```python
from build123d import *

# Parameters (mm, degrees)
SKETCH_R        = 6.2
SKETCH_R_2      = 4
PAD_DEPTH       = 8
PAD001_DEPTH    = 3
FILLET_R        = 1.5
FILLET001_R     = 1
SKETCH002_W     = 2
SKETCH002_H     = 10
SKETCH002_W_2   = 10
SKETCH002_H_2   = 2
PAD002_DEPTH    = 2
CHAMFER_SIZE    = 1.99
SKETCH003_R     = 6.2
SKETCH003_R_2   = 5.59
POCKET_DEPTH    = 3
SKETCH004_W     = 1
SKETCH004_H     = 14
POCKET001_DEPTH = 6
CHAMFER001_SIZE = 0.59
CHAMFER004_SIZE = 1


with BuildPart() as part:
    # Sketch → Pad (new body)
    with BuildSketch(Plane.XY):
        with Locations((15, 15)):
            Circle(SKETCH_R)
        with Locations((15, 15)):
            Circle(SKETCH_R_2, mode=Mode.SUBTRACT)
    extrude(amount=PAD_DEPTH)

    # Sketch001 (on Face3 of Pad) → Pad001 (join)
    with BuildSketch(Plane(origin=(0, 0, 0), x_dir=(1, 0, 0), z_dir=(0, 0, -1))):
        with BuildLine():
            Line((0, -28.504743), (0, 0))
            Line((0, 0), (28.504743, 0))
            ThreePointArc((30.002374, -1.584264), (29.594788, -0.469562), (28.504743, 0))
            ThreePointArc((1.584264, -30.002374), (21.216341, -21.216341), (30.002374, -1.584264))
            ThreePointArc((0, -28.504743), (0.469562, -29.594788), (1.584264, -30.002374))
        make_face()
    extrude(amount=PAD001_DEPTH)

    # Fillet
    fillet_edges = [part.edges().sort_by_distance(p)[0] for p in [
        (0, 0, -1.5),
    ]]
    fillet(fillet_edges, radius=FILLET_R)

    # Fillet001
    fillet001_edges = [part.edges().sort_by_distance(p)[0] for p in [
        (0, 15.002371, -3),
        (0.43934, 0.43934, -3),
        (0.469562, 29.594788, -3),
        (15.002371, 0, -3),
        (21.216341, 21.216341, -3),
        (29.594788, 0.469562, -3),
    ]]
    fillet(fillet001_edges, radius=FILLET001_R)

    # Sketch002 (on Face4 of Fillet001) → Pad002 (join)
    with BuildSketch(Plane.XY):
        with Locations((6, 15)):
            Rectangle(SKETCH002_W, SKETCH002_H)
        with Locations((15, 6)):
            Rectangle(SKETCH002_W_2, SKETCH002_H_2)
    extrude(amount=PAD002_DEPTH)

    # Chamfer
    chamfer_edges = [part.edges().sort_by_distance(p)[0] for p in [
        (15, 5, 0),
        (5, 15, 0),
    ]]
    chamfer(chamfer_edges, length=CHAMFER_SIZE)

    # Sketch003 → Pocket (cut)
    with BuildSketch(Plane.XY):
        with Locations((15, 15)):
            Circle(SKETCH003_R)
        with Locations((15, 15)):
            Circle(SKETCH003_R_2, mode=Mode.SUBTRACT)
    extrude(amount=POCKET_DEPTH, mode=Mode.SUBTRACT)

    # Sketch004 (on Face32 of Pocket) → Pocket001 (cut)
    with BuildSketch(Plane.XY.offset(8)):
        with Locations((15, 15)):
            Rectangle(SKETCH004_W, SKETCH004_H)
    extrude(amount=-POCKET001_DEPTH, mode=Mode.SUBTRACT)

    # Chamfer001
    chamfer001_edges = [part.edges().sort_by_distance(p)[0] for p in [
        (19.557412, 19.20357, 8),
        (19.125718, 18.77181, 3),
        (9.41, 15, 3),
        (9.41, 15, 0),
        (8.8, 15, 8),
    ]]
    chamfer(chamfer001_edges, length=CHAMFER001_SIZE)

    # Chamfer004
    chamfer004_edges = [part.edges().sort_by_distance(p)[0] for p in [
        (11, 15, 0),
    ]]
    chamfer(chamfer004_edges, length=CHAMFER004_SIZE)


solid = part.part
```
The model under review builds one solid part; all positions refer to its coordinate system, in mm. A direction names the side the tool comes from. Round coordinates to 2 decimals unless told otherwise and drop trailing zeros. Loops run counter-clockwise (first coordinate to the right, second up) from the corner with the lowest first, then second, coordinate; pieces in that order, holes last. Notation, with made-up numbers: (86, 4.25) -> (118, 4.25) arc R33 ccw to (118, 41.25) -> close; hole circle Ø2 at (-33, -18). An arc over 180 degrees is marked (long way). Answer as a JSON object with one key per item and string values. Group by question number.
1) For faces 4 (the face through (21.2, 14.9, 5.2)), 5 (the face through (20, 5, 1)), 6 (the face through (7, 15, 1)), 7 (the face through (10, 5, 1)), list the 3-axis set-ups (+Z, -Z, +X, -X, +Y, -Y) from which the entire face can be reached by the end or side of a thin tool; tool diameter is ignored.
2) We need section A-A on z = 4. Write out the cut boundary in (x, y).
3) Mouldability with a two-part tool opening along Z and no side actions: class faces 1 (the face through (20.76, 14.88, 2.58)), 2 (the face through (14.5, 10, 5)), 3 (the face through (10.8, 15.1, 8)) as released by +Z, released by -Z, zero draft, split by the parting line, or undercut.
4) For line 1 (X direction, y = 15, z = 4.25); line 2 (X direction, y = 16, z = 0.25); line 3 (Z direction, x = 26, y = 6), list the stretches that pass through material, from the lowest coordinate up. Write a range as [from, to].
5) For pin 1 Ø2 at (y, z) = (4, 1.5) entering from -X; pin 2 Ø0.6 at (x, y) = (13, 6) entering from +Z; pin 3 Ø1.5 at (x, z) = (9.5, 5) entering from +Y, all flat-tipped, find the tip position at first contact; note any pin that passes through.
Result set:
{
 "1": {"face 4": "+Z, +X", "face 5": "+Z, +X, -Y", "face 6": "+Z, +Y, -Y", "face 7": "+Z, -X, -Y"},
 "2": {"outline": "(14.5, 8.82) -> (14.5, 11.03) arc R4 cw to (14.5, 18.97) -> (14.5, 21.18) arc R6.2 ccw to start; (15.5, 8.82) arc R6.2 ccw to (15.5, 21.18) -> (15.5, 18.97) arc R4 cw to (15.5, 11.03) -> close"},
 "3": {"face 1": "undercut", "face 2": "zero draft", "face 3": "released by +Z"},
 "4": {"line 1": "[8.8, 11], [19, 21.2]", "line 2": "[3.26, 7], [9.15, 11.91], [18.09, 20.85]", "line 3": "[-3, 0]"},
 "5": {"pin 1": "x = 10", "pin 2": "z = 2", "pin 3": "y = 18.98"}
}
